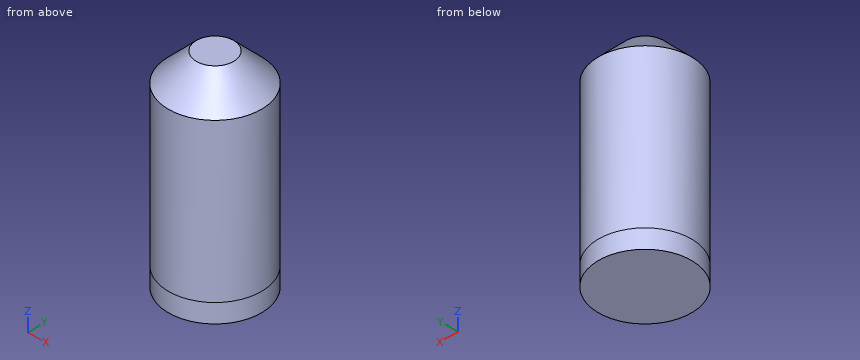
Autodesk Inventor part; units mm, degrees
ref_plane "YZ Plane" through (0, 0, 0) normal (1, 0, 0) x (0, 1, 0)
ref_plane "XZ Plane" through (0, 0, 0) normal (0, 1, 0) x (-1, 0, 0)
ref_plane "XY Plane" through (0, 0, 0) normal (0, 0, 1) x (1, 0, 0)
ref_plane "Work Plane3" through (0, 0, 30) normal (0, 0, 1) x (1, 0, 0)
sketch "Sketch2" plane through (0, 0, 30) normal (0, 0, 1) x (1, 0, 0)
  arc A0 (80, 65) -> (65, 80) centre (65, 65) ccw
  line L0 (80, 65) -> (80, -65)
  arc A1 (65, -80) -> (80, -65) centre (65, -65) ccw
  line L1 (65, -80) -> (-65, -80)
  arc A2 (-80, -65) -> (-65, -80) centre (-65, -65) ccw
  line L2 (-80, -65) -> (-80, 65)
  arc A3 (-65, 80) -> (-80, 65) centre (-65, 65) ccw
  line L3 (-65, 80) -> (65, 80)
  line L4 (-150, -150) -> (150, -150)
  line L5 (150, -150) -> (150, 150)
  line L6 (150, 150) -> (-150, 150)
  line L7 (-150, 150) -> (-150, -150)
  circle A4 centre (0, 0) radius 10
  circle A5 centre (-67, -107.5) radius 1.95
  circle A6 centre (67, 107.5) radius 1.95
  circle A7 centre (-67, 107.5) radius 1.95
  circle A8 centre (67, -107.5) radius 1.95
  dimension "d0" = 20
extrude "Extrusion1" add sketch "Sketch2" along normal blind 40 contours A4
chamfer "Chamfer2" distance 6 angle 45 1 edges at (-10, 0, 70)
sketch "Sketch3" plane through (0, 0, 30) normal (0, 0, -1) x (-1, 0, 0)
  circle A0 centre (0, 0) radius 10
  circle A1 centre (0, 0) radius 10
  dimension "d9" = 20
extrude "Extrusion2" add sketch "Sketch3" along normal blind 4
properties part number "00_Microscope_Objective"
The listing builds one solid part. Answer for the finished solid, in the listing's coordinates (mm). Coordinates: 2 decimals unless noted, no trailing zeros. Loops run counter-clockwise (first coordinate to the right, second up) from the corner with the lowest first, then second, coordinate; pieces in that order, holes last. Notation, with made-up numbers: M 59.25,0.5 L 81.25,0.5 A21 cw 81.25,8.5 Z; hole C 71.5,41.25 d6. An arc over 180 degrees is marked long. Answer as a JSON object with one key per item and string values. Group by question number.
Item 1: Section C-C (z = 41.5) is taken. Write down the section's boundary in (x, y), and give its area (3 significant figures).
Item 2: Section A-A (x = 0) is taken. Write down the section's boundary in (y, z).
Item 3: Each of these flat-tipped pins is pushed along its axis until it touches: P1, Ø1, axis at y = -6, z = 50.5, coming from the -X side; P2, Ø8, axis at x = 5.5, z = 48.5, coming from the -Y side; P3, Ø10, axis at x = 5.5, z = 40.5, coming from the +Y side. Where does it stop, or does it pass through?
Item 4: Section D-D (z = 67) is taken. Write down the section's boundary in (x, y).
Item 5: Consider L1, parallel to Y at x = -0.25, z = 34.5; L2, parallel to X at y = -5.5, z = 29.5; L3, parallel to Z at x = 6.5, y = -1.75. Determine where each line is inside the solid, lowest interval first.
Solved:
{
 "1": {"outline": "C 0,0 d20", "area": "314 mm2"},
 "2": {"outline": "M -10,26 L 10,26 L 10,64 L 4,70 L -4,70 L -10,64 Z"},
 "3": {"P1": "stops at x = -8.35", "P2": "stops at y = -9.89", "P3": "stops at y = 9.99"},
 "4": {"outline": "C 0,0 d14"},
 "5": {"L1": "y = -10 to 10", "L2": "x = -8.35 to 8.35", "L3": "z = 26 to 67.27"}
}
